from build123d import *

# Parameters (mm, degrees)
F0_R     = 10.9982
F1_DEPTH = 12.7


with BuildPart() as f1:
    # F0 (on Top) → F1 (new body)
    with BuildSketch(Plane.XY):
        with BuildLine():
            ThreePointArc((-12.8911538343, 23.1309812626), (0.1344337077, 14.5448476662), (12.9923672765, 23.3800706565))
            ThreePointArc((12.9923672765, 23.3800706565), (13.7234155889, 25.9010103246), (13.97, 28.5142008215))
            ThreePointArc((13.97, 28.5142008215), (-2.7451303188, 42.2118341767), (-12.8911538343, 23.1309812626))
        make_face()
        with Locations((0, 28.5142008215)):
            Circle(F0_R, mode=Mode.SUBTRACT)
        with BuildLine():
            ThreePointArc((22.2838142213, -10.6272858301), (17.3886665619, 0.4495282156), (22.9861698039, 11.1885336382))
            ThreePointArc((22.9861698039, 11.1885336382), (14.477603867, 14.4056755038), (12.9923672765, 23.3800706565))
            ThreePointArc((12.9923672765, 23.3800706565), (0.1344337077, 14.5448476662), (-12.8911538343, 23.1309812626))
            ThreePointArc((-12.8911538343, 23.1309812626), (-13.4224968925, 14.6502977979), (-18.2472138965, 7.6555552505))
            ThreePointArc((-18.2472138965, 7.6555552505), (-16.5460943978, 3.9945583246), (-15.9628193069, 0))
            ThreePointArc((-15.9628193069, 0), (-17.2599076539, -5.8786231583), (-20.9103082456, -10.6656080065))
            ThreePointArc((-20.9103082456, -10.6656080065), (-14.446049098, -11.7957961727), (-10.5239803599, -17.0571028955))
            ThreePointArc((-10.5239803599, -17.0571028955), (-7.90695155, -14.7274286335), (-4.7925511239, -13.1222084165))
            ThreePointArc((-4.7925511239, -13.1222084165), (-8.0065273621, 11.4479875786), (13.97, 0))
            ThreePointArc((13.97, 0), (11.4479875786, -8.0065273621), (4.7925511239, -13.1222084165))
            ThreePointArc((4.7925511239, -13.1222084165), (9.4100623481, -15.9191262024), (12.6223312654, -20.257961001))
            ThreePointArc((12.6223312654, -20.257961001), (14.9684584098, -12.9500609929), (22.2838142213, -10.6272858301))
        make_face()
        with BuildLine():
            ThreePointArc((44.0738063138, -5.7707969136), (44.3558518724, -2.8915228992), (44.45, 0))
            ThreePointArc((44.45, 0), (44.3558518724, 2.8915228992), (44.0738063138, 5.7707969136))
            ThreePointArc((44.0738063138, 5.7707969136), (34.8276475911, 13.5305885528), (22.9861698039, 11.1885336382))
            ThreePointArc((22.9861698039, 11.1885336382), (17.3886665619, 0.4495282156), (22.2838142213, -10.6272858301))
            ThreePointArc((22.2838142213, -10.6272858301), (34.3904586495, -13.6354397899), (44.0738063138, -5.7707969136))
        make_face()
        with Locations((31.3514322042, 0)):
            Circle(F0_R, mode=Mode.SUBTRACT)
        with BuildLine():
            ThreePointArc((-15.9628193069, 0), (-16.5460943978, 3.9945583246), (-18.2472138965, 7.6555552505))
            ThreePointArc((-18.2472138965, 7.6555552505), (-43.7575354965, 2.0095079688), (-20.9103082456, -10.6656080065))
            ThreePointArc((-20.9103082456, -10.6656080065), (-17.2599076539, -5.8786231583), (-15.9628193069, 0))
        make_face()
        with Locations((-29.9328193069, 0)):
            Circle(F0_R, mode=Mode.SUBTRACT)
        with BuildLine():
            ThreePointArc((13.5840434167, -22.9833335078), (12.9846567282, -21.6624735847), (12.6223312654, -20.257961001))
            ThreePointArc((12.6223312654, -20.257961001), (9.4100623481, -15.9191262024), (4.7925511239, -13.1222084165))
            ThreePointArc((4.7925511239, -13.1222084165), (0, -13.97), (-4.7925511239, -13.1222084165))
            ThreePointArc((-4.7925511239, -13.1222084165), (-7.90695155, -14.7274286335), (-10.5239803599, -17.0571028955))
            ThreePointArc((-10.5239803599, -17.0571028955), (-4.9061642029, -39.3245717561), (13.97, -26.2444168329))
            ThreePointArc((13.97, -26.2444168329), (13.873175313, -24.6024951739), (13.5840434167, -22.9833335078))
        make_face()
        with Locations((0, -26.2444168329)):
            Circle(F0_R, mode=Mode.SUBTRACT)
        with BuildLine():
            ThreePointArc((-4.7925511239, -13.1222084165), (0, -13.97), (4.7925511239, -13.1222084165))
            ThreePointArc((4.7925511239, -13.1222084165), (0, -12.2744168329), (-4.7925511239, -13.1222084165))
        make_face()
        with BuildLine():
            ThreePointArc((-4.7925511239, -13.1222084165), (0, -12.2744168329), (4.7925511239, -13.1222084165))
            ThreePointArc((4.7925511239, -13.1222084165), (11.4479875786, -8.0065273621), (13.97, 0))
            ThreePointArc((13.97, 0), (-8.0065273621, 11.4479875786), (-4.7925511239, -13.1222084165))
        make_face()
        Circle(F0_R, mode=Mode.SUBTRACT)
        with BuildLine():
            ThreePointArc((44.0738063138, 5.7707969136), (44.3558518724, 2.8915228992), (44.45, 0))
            ThreePointArc((44.45, 0), (44.3558518724, -2.8915228992), (44.0738063138, -5.7707969136))
            ThreePointArc((44.0738063138, -5.7707969136), (45.005963802, -2.9520614569), (45.3214322042, 0))
            ThreePointArc((45.3214322042, 0), (45.005963802, 2.9520614569), (44.0738063138, 5.7707969136))
        make_face()
    extrude(amount=F1_DEPTH)


solid = f1.part
Can you work these out from the model? Positions are in its coordinate system, mm. A direction names the side the tool comes from. Coordinates: 2 decimals unless noted, no trailing zeros. Order: outer loops, then holes, each group sorted by start corner. A loop starts at its lowest first (then second) coordinate and runs counter-clockwise, first axis right, second up. Notation, with made-up numbers: (3, -19) - (33, -19) arc R9 cw to (33, -2) - close; hole circle Ø3 at (-27.5, -9.5). An arc over 180 degrees is marked (long way). Answer as a JSON object with one key per item and string values. Group by question number.
Q1. I need wall thicknesses on line 1 (Y direction, x = 0, z = 6.75); line 2 (Y direction, x = 31, z = 10.5); line 3 (X direction, y = 4.5, z = 6.5). Which ranges of each line are inside material? Lowest first, please. Write a range as from..to.
Q2. We'd pull the mould along Y, two halves only. Please class faces 3 (the face through (10, -5, 0)), 4 (the face through (-1.43, -15.34, 6.26)): +Y half, -Y half, draft (parallel to the pull), parting line (faces both ways), or undercut.
Q3. Will these pins go through, and if not, where does the flat tip stop? P1, Ø2, axis at x = 4.5, z = 1.5, coming from the +Y side; P2, Ø17.5, axis at x = 0, y = 0, coming from the -Z side; P3, Ø1.5, axis at y = -20.5, z = 3, coming from the +X side; P4, Ø4, axis at y = 18.5, z = 7, coming from the -X side.
Q4. Imagine slicing it at D-D (z = 6). Please give me the cut outline in (x, y).
Q5. Imagine slicing it at C-C (x = -38). Please give me the cut outline in (y, z).
Q6. Imagine slicing it at A-A (x = 0). Please give me the cut outline in (y, z).
Q7. Imagine slicing it at B-B (y = 4). Please give me the cut outline in (x, z), and give its area (3 significant figures).
Q8. On a 3-axis mill with a long thin cutter (end or side, diameter ignored), from which of +Z, -Z, +X, -X, +Y, -Y can I reach the whole of each face in a straight line? I mean faces 1 (the face through (14.563, 14.303, 6.261)), 2 (the face through (10, -5, 12.7)). Say none if no direction works.
Determined:
{
 "1": {"line 1": "y = -40.21..-37.24, -15.25..-11, 11..17.52, 39.51..42.48", "line 2": "y = -13.97..-10.99, 10.99..13.97", "line 3": "x = -43.16..-39.97, -19.9..-10.04, 10.04..21.32, 41.39..44.58"},
 "2": {"face 3": "draft", "face 4": "undercut"},
 "3": {"P1": "stops at y = 42.04", "P2": "passes through", "P3": "stops at x = 12.85", "P4": "stops at x = -12.91"},
 "4": {"outline": "(-20.91, -10.67) arc R8.88 cw to (-10.52, -17.06) arc R13.97 ccw (long way) to (13.58, -22.98) arc R8.37 cw to (22.28, -10.63) arc R13.97 ccw (long way) to (22.99, 11.19) arc R9.11 cw to (12.99, 23.38) arc R13.97 ccw (long way) to (-12.89, 23.13) arc R15.89 cw to (-18.25, 7.66) arc R13.97 ccw (long way) to start; hole circle Ø22 at (-29.93, 0); hole circle Ø22 at (0, -26.24); hole circle Ø22 at (0, 0); hole circle Ø22 at (0, 28.51); hole circle Ø22 at (31.35, 0)"},
 "5": {"outline": "(-11.41, 0) - (-7.48, 0) - (-7.48, 12.7) - (-11.41, 12.7) - close; (7.48, 0) - (11.41, 0) - (11.41, 12.7) - (7.48, 12.7) - close"},
 "6": {"outline": "(-40.21, 0) - (-37.24, 0) - (-37.24, 12.7) - (-40.21, 12.7) - close; (-15.25, 0) - (-11, 0) - (-11, 12.7) - (-15.25, 12.7) - close; (11, 0) - (17.52, 0) - (17.52, 12.7) - (11, 12.7) - close; (39.51, 0) - (42.48, 0) - (42.48, 12.7) - (39.51, 12.7) - close"},
 "7": {"outline": "(-43.32, 0) - (-40.18, 0) - (-40.18, 12.7) - (-43.32, 12.7) - close; (-19.69, 0) - (-10.25, 0) - (-10.25, 12.7) - (-19.69, 12.7) - close; (10.25, 0) - (21.11, 0) - (21.11, 12.7) - (10.25, 12.7) - close; (41.6, 0) - (44.74, 0) - (44.74, 12.7) - (41.6, 12.7) - close", "area": "338 mm2"},
 "8": {"face 1": "+Z, -Z", "face 2": "+Z, +X, -X, +Y, -Y"}
}
